Design review of the part built by this model. Coordinates are the model's own, in mm. Face numbers are marked on the shaded views. Round coordinates to 2 decimals unless told otherwise and drop trailing zeros. Use a Markdown table: item, result.
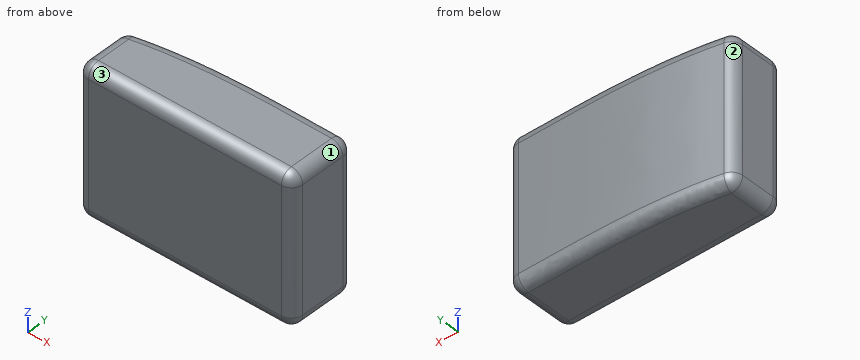
from build123d import *

# Parameters (mm, degrees)
BOSS_EXTRUDE1_DEPTH = 65
FILLET1_R           = 5


with BuildPart() as part:
    # Sketch1 → Boss-Extrude1 (new body)
    with BuildSketch(Plane.XY):
        with BuildLine():
            Line((-42.5, -17), (42.5, -17))
            ThreePointArc((42.5, -17), (46.035533906, -15.535533906), (47.5, -12))
            Line((47.5, -12), (47.5, 8.010433268))
            ThreePointArc((47.5, 8.010433268), (46.0423765, 11.539111311), (42.519372507, 13.010395738))
            add(Edge.make_bspline(
                [(-43.555532841, 7.899733163), (-30.176694997, 10.789213784), (-1.352486938, 13.578958487), (27.425027944, 13.068879237), (42.519372507, 13.010395738)],
                knots=[0.042375719, 0.042375719, 0.042375719, 0.042375719, 0.472818051, 0.947722656, 0.947722656, 0.947722656, 0.947722656], degree=3))
            ThreePointArc((-43.555532841, 7.899733163), (-46.390865213, 6.152667561), (-47.5, 3.012417906))
            Line((-47.5, 3.012417906), (-47.5, -12))
            ThreePointArc((-47.5, -12), (-46.035533906, -15.535533906), (-42.5, -17))
        make_face()
    extrude(amount=BOSS_EXTRUDE1_DEPTH)

    # Fillet1
    fillet1_edges = [part.edges().sort_by_distance(p)[0] for p in [
        (-47.5, -4.493791047, 65),
        (-46.390865213, 6.152667561, 0),
        (-0.682392831, 12.779176888, 0),
        (-46.035533906, -15.535533906, 65),
        (0, -17, 65),
        (46.035533906, -15.535533906, 65),
        (47.5, -1.994783366, 65),
        (46.0423765, 11.539111311, 65),
        (-0.682392831, 12.779176888, 65),
        (-46.390865213, 6.152667561, 65),
        (46.0423765, 11.539111311, 0),
        (47.5, -1.994783366, 0),
        (46.035533906, -15.535533906, 0),
        (0, -17, 0),
        (-46.035533906, -15.535533906, 0),
        (-47.5, -4.493791047, 0),
    ]]
    fillet(fillet1_edges, radius=FILLET1_R)


solid = part.part
1. Wall thickness on line 1 along Y through (x, z) = (39.5, 60); line 2 along X through (y, z) = (7.5, 46.5); line 3 along Z through (x, y) = (-16, -13): over which ranges is each line inside the solid? List them lowest first. Write a range as from..to.
Check values:
| item | result |
|---|---|
| line 1 | y = -17..13.02 |
| line 2 | x = -44.7..47.5 |
| line 3 | z = 0.1..64.9 |
2. The part is to be moulded in two halves that separate along X. For the marked faces 1, 2 and 3, say which applies: pulls with the +X half, pulls with the -X half, needs draft (parallel to the pull), parting line crosses it, or undercut.
Check values:
| item | result |
|---|---|
| face 1 | pulls with the +X half |
| face 2 | pulls with the -X half |
| face 3 | needs draft |
3. Insertion check: pin 1 (3 mm diameter, centred on x = 16.5, z = 24, fed in from +Y). The pin has a flat end and moves straight along its axis. Give the tip position at first contact, or say it passes through.
Check values:
| item | result |
|---|---|
| pin 1 | stops at y = 13.11 |
